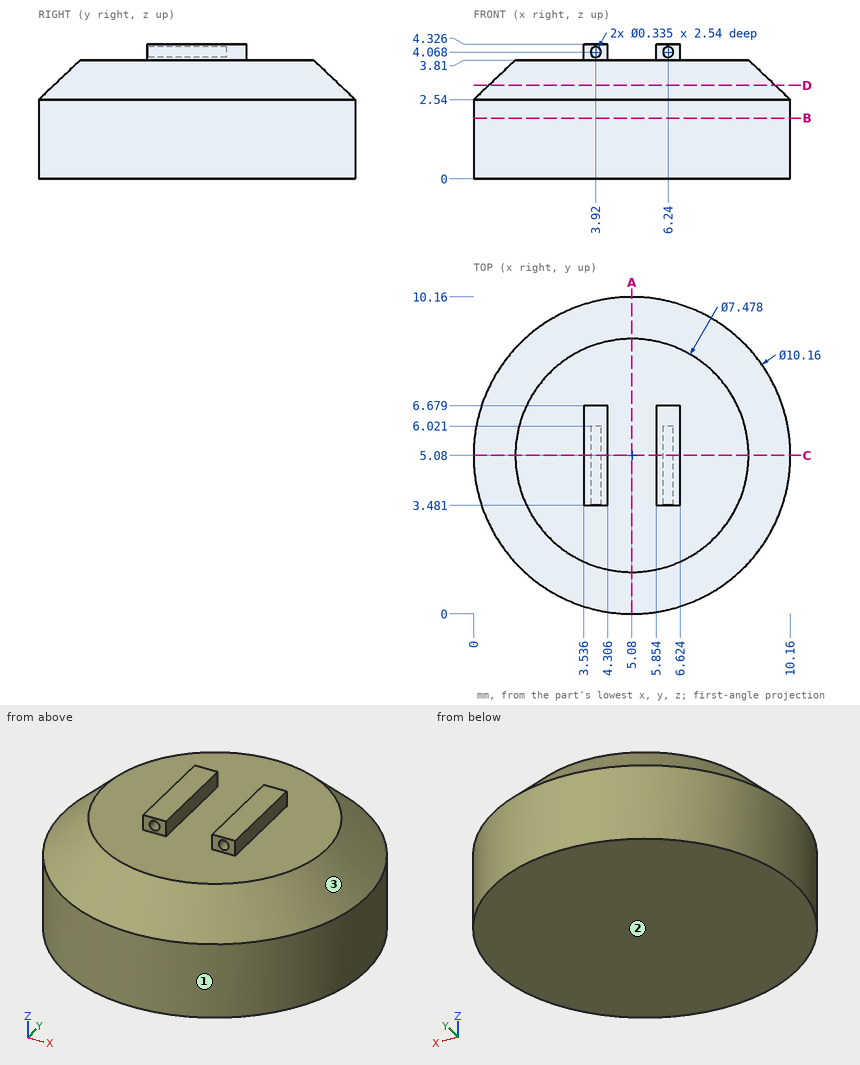
Could you check a few things on this drawing? It's one solid part, dimensions in mm from its lowest x, y, z. Round coordinates to 2 decimals unless told otherwise and drop trailing zeros. Loops run counter-clockwise (first coordinate to the right, second up) from the corner with the lowest first, then second, coordinate; pieces in that order, holes last. Notation, with made-up numbers: M 20.25,14.25 L 53.25,14.25 A18 ccw 53.25,24.25 Z; hole C -21.75,-29 d4. An arc over 180 degrees is marked long. Write item = value, one per line. Start each with the question number.
(1) If we mould it in two halves opening along Z, with no side actions, what happens to the marked faces 1, 2 and 3? For each: released by +Z, released by -Z, zero draft, split by the parting line, or undercut.
(2) I need wall thicknesses on line 1 along Y through (x, z) = (5.25, 1.3); line 2 along Z through (x, y) = (4.75, 6.25); line 3 along Y through (x, z) = (4.25, 2.6). Which ranges of each line are inside material? Lowest first, please.
(3) Suppose I cut it at C-C on y = 5.08. Give the number of separate pieces and of enclosed holes in the cut face, plus the area to 3 significant figures.
(4) Suppose I cut it at B-B on z = 1.95. Write out the boundary of the cut face in (x, y).
(5) I'm going to push flat-ended pins straight in: P1, Ø2, axis at x = 5, y = 9, coming from the +Z side; P2, Ø4, axis at x = 5.5, y = 8, coming from the +Z side. Where does each tip first touch, or does it pass through?
(6) Suppose I cut it at D-D on z = 3. Write out the boundary of the cut face in (x, y).
(7) Suppose I cut it at A-A on x = 5.08. Write out the boundary of the cut face in (y, z).
Answer block:
q1.face_1 = zero draft
q1.face_2 = released by -Z
q1.face_3 = released by +Z
q2.line_1 = 0 to 10.16
q2.line_2 = 0 to 3.81
q2.line_3 = 0.13 to 10.03
q3.separate_pieces = 1
q3.enclosed_holes = 2
q3.area = 37.6 mm²
q4.outline = C 5.08,5.08 d10.16
q5.P1 = 3.81
q5.P2 = 4.33
q6.outline = C 5.08,5.08 d9.19
q7.outline = M 0,0 L 10.16,0 L 10.16,2.54 L 8.82,3.81 L 1.34,3.81 L 0,2.54 Z
